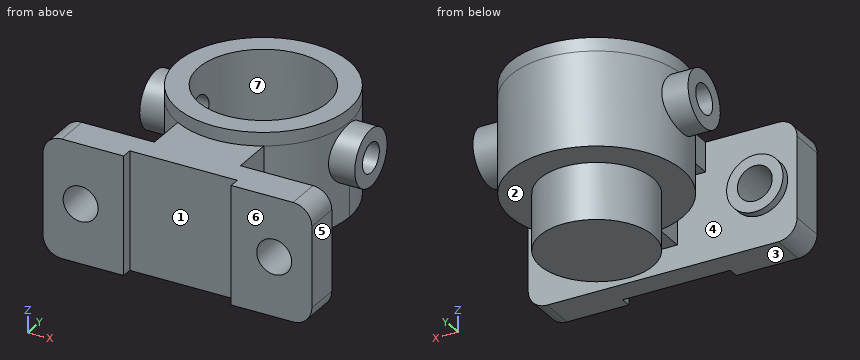
from build123d import *

# Parameters (mm, degrees)
EXTRUDE_1_DEPTH      = 13
SKETCH_2_R           = 10.5
EXTRUDE_2_DEPTH      = 3
EXTRUDE_3_DEPTH      = 56
SKETCH_4_R           = 32
EXTRUDE_4_DEPTH      = 5
EXTRUDE_4_DEPTH_BACK = 35
SKETCH_5_R           = 21
EXTRUDE_5_DEPTH      = 21
SKETCH_6_R           = 10.5
EXTRUDE_6_DEPTH      = 40
SKETCH_7_R           = 5.5
CUT_EXTRUDE_1_DEPTH  = 91
SKETCH_8_R           = 24
CUT_EXTRUDE_2_DEPTH  = 32
SKETCH_9_R           = 12
CUT_EXTRUDE_3_DEPTH  = 21
SKETCH_10_R          = 6.5
CUT_EXTRUDE_4_DEPTH  = 17
SKETCH_11_W          = 40
SKETCH_11_H          = 8
CUT_EXTRUDE_5_DEPTH  = 57


with BuildPart() as part:
    # 草图1 → 凸台-拉伸1 (new body)
    with BuildSketch(Plane(origin=(0, 0, 0), x_dir=(1, 0, 0), z_dir=(0, 1, 0))):
        with BuildLine():
            Line((-43, -22), (43, -22))
            ThreePointArc((43, -22), (47.949747468, -19.949747468), (50, -15))
            Line((50, -15), (50, 15))
            ThreePointArc((50, 15), (47.949747468, 19.949747468), (43, 22))
            Line((43, 22), (-43, 22))
            ThreePointArc((-43, 22), (-47.949747468, 19.949747468), (-50, 15))
            Line((-50, 15), (-50, -15))
            ThreePointArc((-50, -15), (-47.949747468, -19.949747468), (-43, -22))
        make_face()
    extrude(amount=EXTRUDE_1_DEPTH)

    # 草图2 → 凸台-拉伸2 (add)
    with BuildSketch(Plane(origin=(0, 13, 0), x_dir=(1, 0, 0), z_dir=(0, 1, 0))):
        with Locations((-36, 0)):
            Circle(SKETCH_2_R)
        with Locations((36, 0)):
            Circle(SKETCH_2_R)
    extrude(amount=EXTRUDE_2_DEPTH)

    # 草图3 → 凸台-拉伸3 (add)
    with BuildSketch(Plane(origin=(0, 13, 0), x_dir=(1, 0, 0), z_dir=(0, 1, 0))):
        Polygon((16, -22), (-16, -22), (-16, -11), (-5.5, -11), (-5.5, 13), (5.5, 13), (5.5, -11), (16, -11), align=None)
    extrude(amount=EXTRUDE_3_DEPTH)

    # 草图4 → 凸台-拉伸4 (add, two sides)
    with BuildSketch(Plane.XY.offset(22)) as extrude_4_sk:
        with Locations((0, 56)):
            Circle(SKETCH_4_R)
    extrude(amount=EXTRUDE_4_DEPTH)
    extrude(extrude_4_sk.sketch, amount=-EXTRUDE_4_DEPTH_BACK)

    # 草图5 → 凸台-拉伸5 (add)
    with BuildSketch(Plane(origin=(0, 0, -13), x_dir=(-1, 0, 0), z_dir=(0, 0, -1))):
        with Locations((0, 56)):
            Circle(SKETCH_5_R)
    extrude(amount=EXTRUDE_5_DEPTH)

    # 草图6 → 凸台-拉伸6 (add)
    with BuildSketch(Plane(origin=(0, 0, 0), x_dir=(0, 0, -1), z_dir=(1, 0, 0))):
        with Locations((-11, 56)):
            Circle(SKETCH_6_R)
    extrude_6 = extrude(amount=EXTRUDE_6_DEPTH)

    # 镜向1: 凸台-拉伸6 across plane
    add(extrude_6.mirror(Plane(origin=(0, 0, 0), x_dir=(0, 0, 1), z_dir=(1, 0, 0))))

    # 草图7 → 切除-拉伸1 (cut, through all)
    with BuildSketch(Plane.ZY.offset(40)):
        with Locations((11, 56)):
            Circle(SKETCH_7_R)
    extrude(amount=-CUT_EXTRUDE_1_DEPTH, mode=Mode.SUBTRACT)

    # 草图8 → 切除-拉伸2 (cut)
    with BuildSketch(Plane.XY.offset(27)):
        with Locations((0, 56)):
            Circle(SKETCH_8_R)
    extrude(amount=-CUT_EXTRUDE_2_DEPTH, mode=Mode.SUBTRACT)

    # 草图9 → 切除-拉伸3 (cut)
    with BuildSketch(Plane.XY.offset(-5)):
        with Locations((0, 56)):
            Circle(SKETCH_9_R)
    extrude(amount=-CUT_EXTRUDE_3_DEPTH, mode=Mode.SUBTRACT)

    # 草图10 → 切除-拉伸4 (cut, through all)
    with BuildSketch(Plane(origin=(0, 16, 0), x_dir=(1, 0, 0), z_dir=(0, 1, 0))):
        with Locations((-36, 0)):
            Circle(SKETCH_10_R)
        with Locations((36, 0)):
            Circle(SKETCH_10_R)
    extrude(amount=-CUT_EXTRUDE_4_DEPTH, mode=Mode.SUBTRACT)

    # 草图11 → 切除-拉伸5 (cut, through all)
    with BuildSketch(Plane.XY.offset(22)):
        Rectangle(SKETCH_11_W, SKETCH_11_H)
    extrude(amount=-CUT_EXTRUDE_5_DEPTH, mode=Mode.SUBTRACT)


solid = part.part
Geometry check sheet. Reference: the model listing, model coordinates, mm. Face numbers are marked on the shaded views. A direction names the side the tool comes from. Give positions to 0.01 mm unless a question says otherwise; leave off trailing zeros. Order: outer loops, then holes, each group sorted by start corner. A loop starts at its lowest first (then second) coordinate and runs counter-clockwise, first axis right, second up.
1. Sectioned sample at B-B (z = -17). Record the boundary of the cut face in (x, y), then the cut area to 3 significant figures.
Completed:
outline: (-49.71, 0) - (-20, 0) - (-20, 4) - (20, 4) - (20, 0) - (49.71, 0) - (49.71, 13) - (-49.71, 13) - close; circle Ø42 at (0, 56); hole circle Ø24 at (0, 56)
area: 2,070 mm2
2. Access from +Z, -Z, +X, -X, +Y, -Y to the whole of each face (thin tool, end or side, straight path). Record for the marked faces 1, 2, 3 and 4.
Completed:
face 1: +Z, -Z, -Y
face 2: -Z
face 3: -Z, +X, -X, -Y
face 4: none
3. Sectioned sample at C-C (x = -17.5). Record the boundary of the cut face in (y, z), then the cut area to 3 significant figures.
Completed:
outline: (4, -22) - (13, -22) - (13, 22) - (4, 22) - close; (29.21, -13) - (44.39, -13) - (44.39, -34) - (67.61, -34) - (67.61, -13) - (82.79, -13) - (82.79, 27) - (72.42, 27) - (72.42, -5) - (39.58, -5) - (39.58, 27) - (29.21, 27) - close
area: 1,980 mm2
4. Draft check along X on the marked faces 5, 6 and 7. Enter one of: pulls with the +X half, pulls with the -X half, needs draft (parallel to the pull), parting line crosses it, or undercut.
Completed:
face 5: pulls with the +X half
face 6: needs draft
face 7: undercut
5. Scan lines: line 1 (Y direction, x = 34, z = 11); line 2 (Z direction, x = 36, y = 11); line 3 (Y direction, x = 0, z = -9.5). Record each from-to range of solid material in increasing order.
Completed:
line 1: y = 0 to 13, 45.5 to 50.5, 61.5 to 66.5
line 2: z = -22 to -6.5, 6.5 to 22
line 3: y = 4 to 44, 68 to 88
6. Sectioned sample at D-D (y = 40). Record the boundary of the cut face in (x, z).
Completed:
outline: (-27.71, -13) - (-13.6, -13) - (-13.6, -34) - (13.6, -34) - (13.6, -13) - (27.71, -13) - (27.71, 27) - (17.89, 27) - (17.89, -5) - (-17.89, -5) - (-17.89, 27) - (-27.71, 27) - close
7. Sectioned sample at A-A (x = -36). Record the boundary of the cut face in (y, z), then the cut area to 3 significant figures.
Completed:
outline: (0, -22) - (13, -22) - (13, -10.5) - (16, -10.5) - (16, -6.5) - (0, -6.5) - close; (0, 6.5) - (16, 6.5) - (16, 10.5) - (13, 10.5) - (13, 22) - (0, 22) - close; circle Ø21 at (56, 11); hole circle Ø11 at (56, 11)
area: 678 mm2
8. Depth check by flat-ended pin: pin 1 (10.5 mm diameter, centred on y = 56.5, z = 9, fed in from -X); pin 2 (12 mm diameter, centred on x = -13.5, y = 15.5, fed in from -Z); pin 3 (6.5 mm diameter, centred on y = 56, z = 11, fed in from +X); pin 4 (5.5 mm diameter, centred on x = 9, y = 23, fed in from -Z). Enter the tip coordinate at first touch or a pass-through.
Completed:
pin 1: stops at x = -40
pin 2: stops at z = -22
pin 3: passes through
pin 4: stops at z = -13
